Design review of the part built by this model. Coordinates are the model's own, in mm. A direction names the side the tool comes from. Coordinates: 2 decimals unless noted, no trailing zeros. Loops run counter-clockwise (first coordinate to the right, second up) from the corner with the lowest first, then second, coordinate; pieces in that order, holes last. Notation, with made-up numbers: (8.25, 5) -> (23.25, 5) arc R24 cw to (23.25, 30) -> close; hole circle Ø5 at (14.5, -22). An arc over 180 degrees is marked (long way). Use CSV: the item, a comma, the result in double quotes.
```python
from build123d import *

# Parameters (mm, degrees)
F0_R      = 13.137742
F1_DEPTH  = 49.784
F1_FACE_W = 49.784
F1_FACE_H = 55.855792


with BuildPart() as f1:
    # F0 (on Front) → F1 (new body)
    with BuildSketch(Plane.XZ):
        with BuildLine():
            Line((25.885448, 34.804828), (-58.201034, 34.804828))
            Line((-58.201034, 34.804828), (-58.201034, -21.050964))
            Line((-58.201034, -21.050964), (25.885448, -21.050964))
            ThreePointArc((25.885448, -21.050964), (53.813344, 6.876932), (25.885448, 34.804828))
        make_face()
        with Locations((25.885448, 6.876932)):
            Circle(F0_R, mode=Mode.SUBTRACT)
    extrude(amount=F1_DEPTH)

    # F1_face (on face) → F2 (revolve)
    with BuildSketch(Plane(origin=(-58.201034, -24.892, 6.876932), x_dir=(0, -1, 0), z_dir=(-1, 0, 0))):
        Rectangle(F1_FACE_W, F1_FACE_H)
    revolve(axis=Axis((25.885448, -24.892, 34.804828), (0, -1, 0)))


solid = f1.part
```
Item 1: Add section B-B (z = -25.5). Give the boundary of the cut face in (x, y).
Checked values:
outline,"(-55.07, -49.78) -> (-32.71, -49.78) -> (-32.71, 0) -> (-55.07, 0) -> close; (84.48, -49.78) -> (106.84, -49.78) -> (106.84, 0) -> (84.48, 0) -> close"
Item 2: Add section D-D (z = 0.5). Give the boundary of the cut face in (x, y).
Checked values:
outline,"(-69.05, -49.78) -> (14.4, -49.78) -> (14.4, 0) -> (-69.05, 0) -> close; (37.37, -49.78) -> (53.08, -49.78) -> (53.08, 0) -> (37.37, 0) -> close; (102.66, -49.78) -> (120.83, -49.78) -> (120.83, 0) -> (102.66, 0) -> close"
Item 3: Add section A-A (x = -26). Give the boundary of the cut face in (y, z), then the cut area to 3 significant figures.
Checked values:
outline,"(-49.78, -51.79) -> (0, -51.79) -> (0, -31.36) -> (-49.78, -31.36) -> close; (-49.78, -21.05) -> (0, -21.05) -> (0, 34.8) -> (-49.78, 34.8) -> close; (-49.78, 100.97) -> (0, 100.97) -> (0, 121.4) -> (-49.78, 121.4) -> close"
area,"4,810 mm^2"
Item 4: To check wall thickness, follow line 1 along Z through (x, y) = (10.5, -19.5); line 2 along Z through (x, y) = (-32.5, -41.5); line 3 along Z through (x, y) = (22.5, -12). State the ranges of each line that lie inside material, in increasing order.
Checked values:
line 1,"-64.96 to -47.86, -21.05 to 34.8, 117.47 to 134.57"
line 2,"-47.55 to -25.71, -21.05 to 34.8, 95.32 to 117.15"
line 3,"-66.09 to -49.21, -21.05 to -5.82, 19.57 to 34.8, 118.82 to 135.7"
Item 5: Machinability: for faces 1 (the face through (-16, -25, 34.805)), 2 (the face through (9, -49.784, 22)), which of the approach directions +Z, -Z, +X, -X, +Y, -Y give a long, thin tool a straight path to every point of the face, cutting with its end or side? Answer none if there is none.
Checked values:
face 1,"+Y, -Y"
face 2,"+Z, -Z, +X, -X, -Y"
Item 6: Clearance check with flat-ended pins moving along their axes: pin 1 (2 mm diameter, centred on y = -9, z = 42.5, fed in from +X); pin 2 (10 mm diameter, centred on x = -27, y = -25, fed in from -Z); pin 3 (2 mm diameter, centred on x = 45.5, y = -10, fed in from +Z). State where each tip first meets the part, or that it passes through.
Checked values:
pin 1,"x = 126.61"
pin 2,"z = -54.06"
pin 3,"z = 134.02"
Item 7: Add section C-C (x = 31). Give the boundary of the cut face in (y, z).
Checked values:
outline,"(-49.78, -66.01) -> (0, -66.01) -> (0, -49.13) -> (-49.78, -49.13) -> close; (-49.78, -20.58) -> (0, -20.58) -> (0, -5.22) -> (-49.78, -5.22) -> close; (-49.78, 18.98) -> (0, 18.98) -> (0, 34.33) -> (-49.78, 34.33) -> close; (-49.78, 118.74) -> (0, 118.74) -> (0, 135.62) -> (-49.78, 135.62) -> close"
